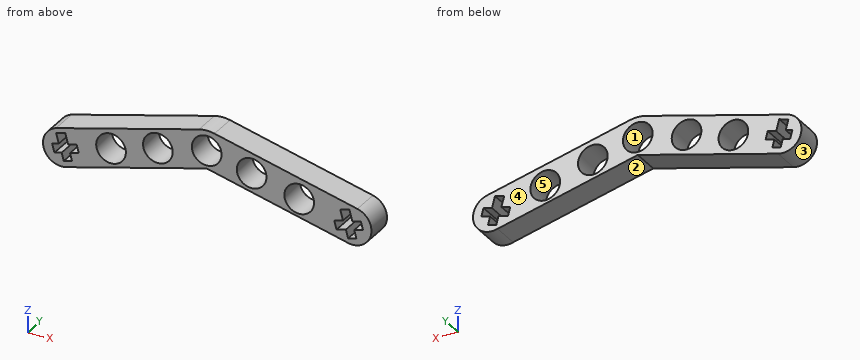
from build123d import *

# Parameters (mm, degrees)
F0_R     = 2.42261
F1_DEPTH = 2.286
F2_R     = 5.08


with BuildPart() as f1:
    # F0 (on Front) → F1 (new body, symmetric)
    with BuildSketch(Plane.XZ):
        with BuildLine():
            Line((0, 6.35), (-24.593444, 0))
            ThreePointArc((-24.593444, 0), (-26.606894, -3.785008), (-22.882334, -5.908193))
            Line((-22.882334, -5.908193), (0, 0))
            Line((0, 0), (22.882336, -5.908194))
            ThreePointArc((22.882336, -5.908194), (26.779601, -3.835026), (24.593444, 0))
            Line((24.593444, 0), (0, 6.35))
        make_face()
        Polygon((-25.233058, -2.70493), (-24.149164, -2.412652), (-24.593444, -0.765068), (-23.096818, -0.361495), (-22.609838, -2.167426), (-21.225002, -1.793997), (-20.880997, -3.069718), (-22.308412, -3.454628), (-21.983574, -4.659269), (-23.335583, -5.023846), (-23.679588, -3.748126), (-24.862724, -4.07829), align=None, mode=Mode.SUBTRACT)
        with Locations((-15.617909, -0.922615)):
            Circle(F0_R, mode=Mode.SUBTRACT)
        Polygon((20.821678, -2.915041), (22.254047, -2.528795), (21.809766, -0.881211), (23.306393, -0.477637), (23.793373, -2.283569), (25.178209, -1.91014), (25.522214, -3.18586), (24.094798, -3.570771), (24.43871, -4.846144), (23.086701, -5.210721), (22.723623, -3.864269), (21.192243, -4.291613), align=None, mode=Mode.SUBTRACT)
        with Locations((15.105182, -0.922615)):
            Circle(F0_R, mode=Mode.SUBTRACT)
        with Locations((-7.967982, 1.174946)):
            Circle(F0_R, mode=Mode.SUBTRACT)
        with Locations((0, 2.902348)):
            Circle(F0_R, mode=Mode.SUBTRACT)
        with Locations((7.33187, 1.174946)):
            Circle(F0_R, mode=Mode.SUBTRACT)
    extrude(amount=F1_DEPTH, both=True)

    # F2
    f2_edges = [f1.edges().sort_by_distance(p)[0] for p in [
        (0, 0, 6.35),
    ]]
    fillet(f2_edges, radius=F2_R)


solid = f1.part
Design review of the part built by this model. Coordinates are the model's own, in mm. Face numbers are marked on the shaded views. A direction names the side the tool comes from. Give positions to 0.01 mm unless a question says otherwise; leave off trailing zeros. Use CSV: the item, a comma, the result in double quotes. Start each with the question number.
1. Draft analysis for pull direction Z (two halves, no side actions). For the marked faces 3, 4 and 5, state which applies: released by +Z, released by -Z, zero draft, split by the parting line, or undercut.
2. Wall thickness on L1, parallel to Z at x = 0, y = -0.45; L2, parallel to Z at x = -15, y = 0.7; L3, parallel to Z at x = 4, y = 1.4: over which ranges is each line inside the solid? List them lowest first.
3. Insertion check: P1, Ø2, axis at x = -9.5, y = 0.5, coming from the -Z side; P2, Ø1.5, axis at y = -1, z = -4.5, coming from the -X side; P3, Ø2, axis at x = 8, y = -0.5, coming from the -Z side. Each pin has a flat end and moves straight along its axis. Give the tip position at first contact, or say it passes through.
4. Machinability: for the marked faces 1 and 2, which of the approach directions +Z, -Z, +X, -X, +Y, -Y give a long, thin tool a straight path to every point of the face, cutting with its end or side? Answer none if there is none.
5. Add section A-A (y = -1.4). Count the separate pieces of the cut face and the enclosed holes in it, plus the area to 3 significant figures.
Results found:
1,face 3,"split by the parting line"
1,face 4,"zero draft"
1,face 5,"undercut"
2,L1,"z = 0 to 0.48, 5.32 to 6.18"
2,L2,"z = -3.87 to -3.27, 1.42 to 2.48"
2,L3,"z = -1.03 to 5.32"
3,P1,"stops at z = -2.71"
3,P2,"stops at x = -26.62"
3,P3,"stops at z = -2.32"
4,face 1,"+Y, -Y"
4,face 2,"-Z, +Y, -Y"
5,separate pieces,"1"
5,enclosed holes,"7"
5,area,"218 mm²"
